Input: part model. Units: mm. Frame: model coordinates. Face numbers are marked on the shaded views. Coordinates: 2 decimals unless noted, no trailing zeros. Order: outer loops, then holes, each group sorted by start corner. A loop starts at its lowest first (then second) coordinate and runs counter-clockwise, first axis right, second up. Notation, with made-up numbers: (5.25, 55.5) -> (31.25, 55.5) arc R14 ccw to (31.25, 62.5) -> close; hole circle Ø9 at (74, -6). An arc over 180 degrees is marked (long way). Use one line per item in the form item = value. Start each with the question number.
1) Draft query along X for the marked faces 1 and 2. Return one class per face: pulls with the +X half, pulls with the -X half, needs draft (parallel to the pull), parting line crosses it, or undercut.
2) Section query B-B on z = 11. Output: boundary loops of the cut face in (x, y).
3) Pin query (flat end, axial travel): pin 1 (12 mm diameter, centred on x = 69, y = -42.5, fed in from -Z); pin 2 (2 mm diameter, centred on x = 20, z = 2, fed in from +Y); pin 3 (8 mm diameter, centred on y = -47.5, z = 8.5, fed in from -X); pin 4 (10 mm diameter, centred on y = 26, z = 3.5, fed in from -X). Return the tip coordinate at first contact, or that it passes through.
4) Ray query, line 1 along Y through (x, z) = (0, 2.05); line 2 along Y through (x, z) = (-81, 16); line 3 along X through (y, z) = (58, 7.5). Return the intervals inside material, ascending.
5) Section query D-D on x = 72. Output: boundary loops of the cut face in (y, z), then the cut area to 3 significant figures.
6) Section query A-A on y = -54. Output: boundary loops of the cut face in (x, z).
7) Section query C-C on x = 47. Output: boundary loops of the cut face in (y, z), then the cut area to 3 significant figures.
from build123d import *

# Parameters (mm, degrees)
SKETCH019_W     = 179.8
SKETCH019_H     = 140
PAD006_DEPTH    = 18
POCKET005_DEPTH = 140.001
SKETCH020_R     = 1.5
POCKET006_DEPTH = 18.001
CHAMFER004_SIZE = 1.8
CHAMFER009_SIZE = 2


with BuildPart() as part:
    # Sketch019 → Pad006 (new body)
    with BuildSketch(Plane.XY):
        Rectangle(SKETCH019_W, SKETCH019_H)
    extrude(amount=PAD006_DEPTH)

    # Sketch017 (on Face3 of Pad006) → Pocket005 (cut, through all)
    with BuildSketch(Plane.XZ.offset(70)):
        with BuildLine():
            Line((-76.9, 18), (76.9, 18))
            Line((76.9, 18), (76.9, 13))
            Line((76.9, 13), (84.9, 13))
            Line((84.9, 13), (84.9, 8))
            ThreePointArc((81.9, 5), (84.0213203436, 5.8786796564), (84.9, 8))
            Line((81.9, 5), (-81.9, 5))
            ThreePointArc((-84.9, 8), (-84.0213203436, 5.8786796564), (-81.9, 5))
            Line((-84.9, 13), (-84.9, 8))
            Line((-76.9, 13), (-84.9, 13))
            Line((-76.9, 18), (-76.9, 13))
        make_face()
    extrude(amount=-POCKET005_DEPTH, mode=Mode.SUBTRACT)

    # Sketch020 (on Face2 of Pocket005) → Pocket006 (cut, through all)
    with BuildSketch(Plane(origin=(0, 0, 0), x_dir=(1, 0, 0), z_dir=(0, 0, -1))):
        with Locations((0, -10)):
            Circle(SKETCH020_R)
        with Locations((0, 10)):
            Circle(SKETCH020_R)
        with BuildLine():
            Line((-75.9, -70), (75.9, -70))
            ThreePointArc((75.9, -70), (0, -42.4418315883), (-75.9, -70))
        make_face()
        with BuildLine():
            Line((75.9, 50), (30.4697456096, 16.0147901872))
            ThreePointArc((30.4697456096, 16.0147901872), (22.45, 0), (30.4697456096, -16.0147901872))
            Line((75.9, -50), (30.4697456096, -16.0147901872))
            Line((75.9, -50), (89.9, -50))
            Line((89.9, 50), (89.9, -50))
            Line((75.9, 50), (89.9, 50))
        make_face()
        with BuildLine():
            ThreePointArc((-30.4697456096, -16.0147901872), (-22.45, 0), (-30.4697456096, 16.0147901872))
            Line((-75.9, 50), (-30.4697456096, 16.0147901872))
            Line((-75.9, 50), (-89.9, 50))
            Line((-89.9, 50), (-89.9, -50))
            Line((-89.9, -50), (-75.9, -50))
            Line((-75.9, -50), (-30.4697456096, -16.0147901872))
        make_face()
        with BuildLine():
            Line((-75.9, 70), (75.9, 70))
            ThreePointArc((-75.9, 70), (0, 42.4418315883), (75.9, 70))
        make_face()
    extrude(amount=-POCKET006_DEPTH, mode=Mode.SUBTRACT)

    # Chamfer004
    chamfer004_edges = [part.edges().sort_by_distance(p)[0] for p in [
        (-1.5, -10, 5),
        (-1.5, 10, 5),
    ]]
    chamfer(chamfer004_edges, length=CHAMFER004_SIZE)

    # Chamfer009
    chamfer009_edges = [part.edges().sort_by_distance(p)[0] for p in [
        (83.4, 70, 18),
        (89.9, 60, 18),
        (83.4, 50, 18),
        (76.9, 60, 18),
        (89.9, 60, 0),
        (89.9, 50, 9),
        (89.9, 70, 9),
        (83.4, -50, 18),
        (89.9, -60, 18),
        (83.4, -70, 18),
        (76.9, -60, 18),
        (89.9, -60, 0),
        (89.9, -70, 9),
        (89.9, -50, 9),
        (-89.9, 60, 0),
        (-89.9, 70, 9),
        (-89.9, 60, 18),
        (-89.9, 50, 9),
        (-89.9, -60, 0),
        (-89.9, -50, 9),
        (-89.9, -60, 18),
        (-89.9, -70, 9),
        (-83.4, -50, 18),
        (-76.9, -60, 18),
        (-83.4, -70, 18),
        (-83.4, 70, 18),
        (-76.9, 60, 18),
        (-83.4, 50, 18),
    ]]
    chamfer(chamfer009_edges, length=CHAMFER009_SIZE)


solid = part.part
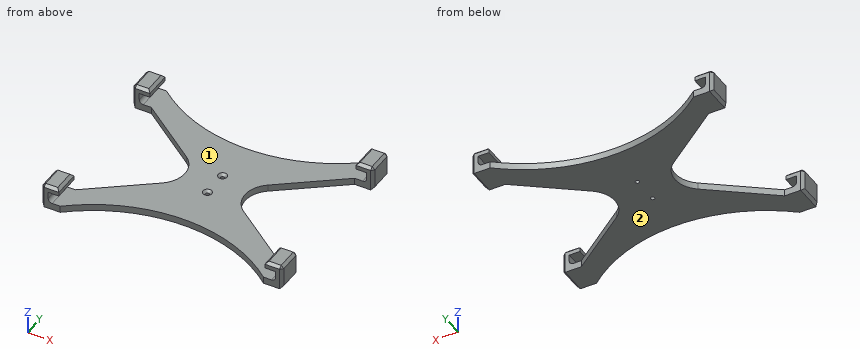
Answers below:
q1.face_1 = undercut
q1.face_2 = needs draft
q2.outline = (-89.9, -68) -> (-87.9, -70) -> (-84.9, -70) -> (-84.9, -50) -> (-87.9, -50) -> (-89.9, -52) -> close; (-89.9, 52) -> (-87.9, 50) -> (-84.9, 50) -> (-84.9, 70) -> (-87.9, 70) -> (-89.9, 68) -> close; (84.9, -70) -> (87.9, -70) -> (89.9, -68) -> (89.9, -52) -> (87.9, -50) -> (84.9, -50) -> close; (84.9, 50) -> (87.9, 50) -> (89.9, 52) -> (89.9, 68) -> (87.9, 70) -> (84.9, 70) -> close
q3.pin_1 = 0
q3.pin_2 = 44.32
q3.pin_3 = -89.4
q3.pin_4 = -50.5
q4.line_1 = -42.44 to -11.5, -8.5 to 8.5, 11.5 to 42.44
q4.line_2 = -70 to -50, 50 to 70
q4.line_3 = -89.9 to -84.86, 84.86 to 89.9
q5.outline = (-66.88, 0) -> (-47.08, 0) -> (-47.08, 5) -> (-66.88, 5) -> close; (47.08, 0) -> (66.88, 0) -> (66.88, 5) -> (47.08, 5) -> close
q5.area = 198 mm^2
q6.outline = (-89.9, 2) -> (-87.9, 0) -> (-51, 0) -> (-51, 5) -> (-81.9, 5) arc R3 cw to (-84.9, 8) -> (-84.9, 13) -> (-76.9, 13) -> (-76.9, 16) -> (-78.9, 18) -> (-87.9, 18) -> (-89.9, 16) -> close; (51, 0) -> (87.9, 0) -> (89.9, 2) -> (89.9, 16) -> (87.9, 18) -> (78.9, 18) -> (76.9, 16) -> (76.9, 13) -> (84.9, 13) -> (84.9, 8) arc R3 cw to (81.9, 5) -> (51, 5) -> close
q7.outline = (-52.18, 0) -> (-28.38, 0) -> (-28.38, 5) -> (-52.18, 5) -> close; (28.38, 0) -> (52.18, 0) -> (52.18, 5) -> (28.38, 5) -> close
q7.area = 238 mm^2
